Can you work these out from the model? Positions are in its coordinate system, mm. A direction names the side the tool comes from. Give positions to 0.01 mm unless a question says otherwise; leave off trailing zeros. Order: outer loops, then holes, each group sorted by start corner. A loop starts at its lowest first (then second) coordinate and runs counter-clockwise, first axis right, second up. Notation, with made-up numbers: (32.25, 80.5) - (44.25, 80.5) arc R16 ccw to (44.25, 102.5) - close; hole circle Ø5 at (-29.5, 65). An arc over 180 degrees is marked (long way). Return JSON: item names as keys, results as strings.
```python
from build123d import *

# Parameters (mm, degrees)
SKETCH1_W               = 450
SKETCH1_H               = 125.6
BOSS_EXTRUDE1_DEPTH     = 1.22
EDGE_FLANGE1_DEPTH      = 450
EDGE_FLANGE1_BEND_DEPTH = 450
CUT_EXTRUDE1_DEPTH      = 265.939058972
CUT_EXTRUDE1_DEPTH_BACK = 265.939058972
CUT_EXTRUDE2_DEPTH      = 266.511236239
CUT_EXTRUDE2_DEPTH_BACK = 266.511236239
SKETCH13_R              = 17.5
SKETCH13_R_2            = 3
CUT_EXTRUDE3_DEPTH      = 265.939058972
CUT_EXTRUDE3_DEPTH_BACK = 265.939058972
CUT_EXTRUDE4_DEPTH      = 265.939058972
CUT_EXTRUDE4_DEPTH_BACK = 265.939058972
SKETCH17_R              = 1.6


# Sheet-metal steps are written as plain solids
with BuildPart() as part:
    # Sketch1 → Boss-Extrude1 (new body)
    with BuildSketch(Plane(origin=(0, 0, 0), x_dir=(1, 0, 0), z_dir=(0, 1, 0))):
        Rectangle(SKETCH1_W, SKETCH1_H)
    extrude(amount=BOSS_EXTRUDE1_DEPTH)

    # Edge-Flange1 section (across the edge) → Edge-Flange1 (add)
    with BuildSketch(Plane(origin=(225, 0, 63.943), x_dir=(0, 0, -1), z_dir=(-1, 0, 0))):
        with BuildLine():
            Line((-1.22, 1.143), (-1.22, 123.78))
            Line((-1.22, 123.78), (0, 123.78))
            Line((0, 123.78), (0, 1.143))
            ThreePointArc((0, 1.143), (0.334776949, 0.334776949), (1.143, 0))
            Line((1.143, 0), (1.143, -1.22))
            ThreePointArc((1.143, -1.22), (-0.527893324, -0.527893324), (-1.22, 1.143))
        make_face()
    extrude(amount=EDGE_FLANGE1_DEPTH)

    # Edge-Flange1 section 2 (across the edge) → Edge-Flange1 bend (add)
    with BuildSketch(Plane(origin=(-225, 0, -63.943), x_dir=(0, 0, 1), z_dir=(1, 0, 0))):
        with BuildLine():
            Line((-1.22, 1.143), (-1.22, 123.78))
            Line((-1.22, 123.78), (0, 123.78))
            Line((0, 123.78), (0, 1.143))
            ThreePointArc((0, 1.143), (0.334776949, 0.334776949), (1.143, 0))
            Line((1.143, 0), (1.143, -1.22))
            ThreePointArc((1.143, -1.22), (-0.527893324, -0.527893324), (-1.22, 1.143))
        make_face()
    extrude(amount=EDGE_FLANGE1_BEND_DEPTH)

    # Sketch12 → Cut-Extrude1 (cut, two sides: drawn at the far end of the back side and taken through both)
    with BuildSketch(Plane.XY.offset(-CUT_EXTRUDE1_DEPTH_BACK)):
        Polygon((225, -3.78), (225, -28.78), (210.508996835, -223.78), (210.508996835, -248.78), (235.508996835, -248.78), (235.508996835, -3.78), align=None)
    extrude(amount=CUT_EXTRUDE1_DEPTH + CUT_EXTRUDE1_DEPTH_BACK, mode=Mode.SUBTRACT)

    # Sketch13 → Cut-Extrude2 (cut, two sides: drawn at the far end of the back side and taken through both)
    with BuildSketch(Plane(origin=(0, 1.22, 0), x_dir=(1, 0, 0), z_dir=(0, 1, 0)).offset(-CUT_EXTRUDE2_DEPTH_BACK)):
        with Locations(Location((150, 0, 0), (0, 0, 270))):
            Circle(SKETCH13_R)
        with Locations(Location((114.948, 7.564, 0), (0, 0, 270))):
            Circle(SKETCH13_R_2)
        with Locations(Location((114.947, -7.548, 0), (0, 0, 270))):
            Circle(SKETCH13_R_2)
        with BuildLine():
            Line((45, 3), (53.205505282, 3))
            ThreePointArc((53.205505282, 3), (97, 0), (53.205505282, -3))
            Line((53.205505282, -3), (45, -3))
            ThreePointArc((45, -3), (42, 0), (45, 3))
        make_face()
        with BuildLine():
            Line((-30, 3), (-21.794494718, 3))
            ThreePointArc((-21.794494718, 3), (22, 0), (-21.794494718, -3))
            Line((-21.794494718, -3), (-30, -3))
            ThreePointArc((-30, -3), (-33, 0), (-30, 3))
        make_face()
        with BuildLine():
            Line((-105, 3), (-96.794494718, 3))
            ThreePointArc((-96.794494718, 3), (-53, 0), (-96.794494718, -3))
            Line((-96.794494718, -3), (-105, -3))
            ThreePointArc((-105, -3), (-108, 0), (-105, 3))
        make_face()
        with BuildLine():
            Line((-180, 3), (-171.794494718, 3))
            ThreePointArc((-171.794494718, 3), (-128, 0), (-171.794494718, -3))
            Line((-171.794494718, -3), (-180, -3))
            ThreePointArc((-180, -3), (-183, 0), (-180, 3))
        make_face()
    extrude(amount=CUT_EXTRUDE2_DEPTH + CUT_EXTRUDE2_DEPTH_BACK, mode=Mode.SUBTRACT)

    # Sketch16 → Cut-Extrude3 (cut, two sides: drawn at the far end of the back side and taken through both)
    with BuildSketch(Plane.XY.offset(-CUT_EXTRUDE3_DEPTH_BACK)):
        with BuildLine():
            Line((-22.5, -104.646), (-167.5, -104.646))
            ThreePointArc((-167.5, -104.646), (-171.035533906, -103.181533906), (-172.5, -99.646))
            Line((-172.5, -99.646), (-172.5, -39.646))
            ThreePointArc((-172.5, -39.646), (-171.035533906, -36.110466094), (-167.5, -34.646))
            Line((-167.5, -34.646), (-22.5, -34.646))
            ThreePointArc((-22.5, -34.646), (-18.964466094, -36.110466094), (-17.5, -39.646))
            Line((-17.5, -39.646), (-17.5, -99.646))
            ThreePointArc((-17.5, -99.646), (-18.964466094, -103.181533906), (-22.5, -104.646))
        make_face()
        with BuildLine():
            Line((172.5, -99.646), (172.5, -39.646))
            ThreePointArc((172.5, -39.646), (171.035533906, -36.110466094), (167.5, -34.646))
            Line((167.5, -34.646), (22.5, -34.646))
            ThreePointArc((22.5, -34.646), (18.964466094, -36.110466094), (17.5, -39.646))
            Line((17.5, -39.646), (17.5, -99.646))
            ThreePointArc((17.5, -99.646), (18.964466094, -103.181533906), (22.5, -104.646))
            Line((22.5, -104.646), (167.5, -104.646))
            ThreePointArc((167.5, -104.646), (171.035533906, -103.181533906), (172.5, -99.646))
        make_face()
    extrude(amount=CUT_EXTRUDE3_DEPTH + CUT_EXTRUDE3_DEPTH_BACK, mode=Mode.SUBTRACT)

    # Sketch17 → Cut-Extrude4 (cut, two sides: drawn at the far end of the back side and taken through both)
    with BuildSketch(Plane.XY.offset(-CUT_EXTRUDE4_DEPTH_BACK)):
        with Locations((-190, -27.4)):
            Circle(SKETCH17_R)
        with Locations((-114, -27.4)):
            Circle(SKETCH17_R)
        with Locations((-38, -27.4)):
            Circle(SKETCH17_R)
        with Locations((38, -27.4)):
            Circle(SKETCH17_R)
        with Locations((114, -27.4)):
            Circle(SKETCH17_R)
        with Locations((190, -27.4)):
            Circle(SKETCH17_R)
        with Locations((190, -117.4)):
            Circle(SKETCH17_R)
        with Locations((114, -117.4)):
            Circle(SKETCH17_R)
        with Locations((38, -117.4)):
            Circle(SKETCH17_R)
        with Locations((-38, -117.4)):
            Circle(SKETCH17_R)
        with Locations((-114, -117.4)):
            Circle(SKETCH17_R)
        with Locations((-190, -117.4)):
            Circle(SKETCH17_R)
    extrude(amount=CUT_EXTRUDE4_DEPTH + CUT_EXTRUDE4_DEPTH_BACK, mode=Mode.SUBTRACT)


solid = part.part
```
1. Suppose I cut it at A-A (x = 150). List the corners of the cut face in (y, z) for me.
Checks:
{"outline": "(-123.78, -65.16) - (-104.65, -65.16) - (-104.65, -63.94) - (-123.78, -63.94) - close; (-123.78, 63.94) - (-104.65, 63.94) - (-104.65, 65.16) - (-123.78, 65.16) - close; (-34.65, -65.16) - (-1.14, -65.16) arc R2.36 ccw to (1.22, -62.8) - (1.22, -17.5) - (0, -17.5) - (0, -62.8) arc R1.14 cw to (-1.14, -63.94) - (-34.65, -63.94) - close; (-34.65, 63.94) - (-1.14, 63.94) arc R1.14 cw to (0, 62.8) - (0, 17.5) - (1.22, 17.5) - (1.22, 62.8) arc R2.36 ccw to (-1.14, 65.16) - (-34.65, 65.16) - close"}
2. Suppose I cut it at B-B (x = 31). List the corners of the cut face in (y, z) for me, plus the area to 3 significant figures.
Checks:
{"outline": "(-123.78, -65.16) - (-104.65, -65.16) - (-104.65, -63.94) - (-123.78, -63.94) - close; (-123.78, 63.94) - (-104.65, 63.94) - (-104.65, 65.16) - (-123.78, 65.16) - close; (-34.65, -65.16) - (-1.14, -65.16) arc R2.36 ccw to (1.22, -62.8) - (1.22, 62.8) arc R2.36 ccw to (-1.14, 65.16) - (-34.65, 65.16) - (-34.65, 63.94) - (-1.14, 63.94) arc R1.14 cw to (0, 62.8) - (0, -62.8) arc R1.14 cw to (-1.14, -63.94) - (-34.65, -63.94) - close", "area": "288 mm^2"}
3. If I drill on L1, parallel to Z at x = 204.5, y = -83.5; L2, parallel to Y at x = -38, z = 64.2; L3, parallel to Y at x = 38, z = -64, over which ranges is the centre line in solid material (lowest first)? Write a range as [from, to].
Checks:
{"L1": "[-65.16, -63.94], [63.94, 65.16]", "L2": "[-123.78, -119], [-115.8, -104.65], [-34.65, -29], [-25.8, 0.76]", "L3": "[-123.78, -119], [-115.8, -104.65], [-34.65, -29], [-25.8, 0.89]"}
4. On a 3-axis mill with a long thin cutter (end or side, diameter ignored), from which of +Z, -Z, +X, -X, +Y, -Y can I reach the whole of each face in a straight line? I mean faces 5 (the face through (-3, -63, -63.943)), 6 (the face through (96.98, 0.6, -0.93)). Say none if no direction works.
Checks:
{"face 5": "+X, -X, -Y", "face 6": "+Y, -Y"}
5. For pin 1 Ø0.6 at (x, y) = (-175, 0.5) entering from -Z; pin 2 Ø12 at (x, z) = (-94, 26.5) entering from -Y; pin 3 Ø1 at (x, y) = (-27, 1) entering from +Z, each with a flat end and sliding along its axis, tell me the tip position at first contact or that it passes through.
Checks:
{"pin 1": "z = -64.74", "pin 2": "y = 0", "pin 3": "z = 64.5"}
6. Thinking about a two-plate mould opening in Z: for faces 1 (the face through (167.35, 0.6, -2.28)), 2 (the face through (3, -48, 65.163)), 3 (the face through (-3, -48, -65.163)), 4 (the face through (-3, 1.22, -29)), which applies, +Z half, -Z half, draft (parallel to the pull), parting line (faces both ways), or undercut?
Checks:
{"face 1": "undercut", "face 2": "+Z half", "face 3": "-Z half", "face 4": "draft"}
7. Suppose I cut it at C-C (y = -18.5). List the corners of the cut face in (x, z) for me.
Checks:
{"outline": "(-225, -65.16) - (225, -65.16) - (225, -63.94) - (-225, -63.94) - close; (-225, 63.94) - (225, 63.94) - (225, 65.16) - (-225, 65.16) - close"}
8. Suppose I cut it at D-D (y = -69.5). List the corners of the cut face in (x, z) for me.
Checks:
{"outline": "(-225, -65.16) - (-172.5, -65.16) - (-172.5, -63.94) - (-225, -63.94) - close; (-225, 63.94) - (-172.5, 63.94) - (-172.5, 65.16) - (-225, 65.16) - close; (-17.5, -65.16) - (17.5, -65.16) - (17.5, -63.94) - (-17.5, -63.94) - close; (-17.5, 63.94) - (17.5, 63.94) - (17.5, 65.16) - (-17.5, 65.16) - close; (172.5, -65.16) - (221.97, -65.16) - (221.97, -63.94) - (172.5, -63.94) - close; (172.5, 63.94) - (221.97, 63.94) - (221.97, 65.16) - (172.5, 65.16) - close"}
